Source: CAD feature listing. Evaluate the final solid. Frame: model axes, mm. Face numbers are marked on the shaded views. A direction names the side the tool comes from. Round coordinates to 2 decimals unless told otherwise and drop trailing zeros. Loops run counter-clockwise (first coordinate to the right, second up) from the corner with the lowest first, then second, coordinate; pieces in that order, holes last. Notation, with made-up numbers: (59.25, 36) -> (117.25, 36) arc R12 cw to (117.25, 52) -> close; hole circle Ø4 at (83.25, -29.75). An arc over 180 degrees is marked (long way). Write item = value, one per line.
from build123d import *

# Parameters (mm, degrees)
CYLINDER002_R               = 27.5
CYLINDER002_DEPTH           = 120
CYLINDER001_R               = 27.5
CYLINDER001_DEPTH           = 120
CYLINDER001_ROLL_ANGLE      = 89.363406
CYLINDER001_PITCH_ANGLE     = 89.363406
CYLINDER001_PLACEMENT_ANGLE = 90
CYLINDER_R                  = 27.5
CYLINDER_DEPTH              = 120
BOX001_W                    = 80
BOX001_H                    = 80
BOX001_DEPTH                = 80
BOX_W                       = 90
BOX_H                       = 90
BOX_DEPTH                   = 90


with BuildPart() as cylinder002:
    # Cylinder002 → Cylinder002 (new body)
    with BuildSketch(Plane.XZ.offset(-60)):
        Circle(CYLINDER002_R)
    extrude(amount=CYLINDER002_DEPTH)


with BuildPart() as cylinder001:
    # Cylinder001 → Cylinder001 (new body)
    with BuildSketch(Plane.XY):
        Circle(CYLINDER001_R)
    extrude(amount=CYLINDER001_DEPTH)


with BuildPart() as cylinder001_1:
    # Cylinder001 roll: moved
    add(cylinder001.part.rotate(Axis((0, 0, 0), (1, 0, 0)), CYLINDER001_ROLL_ANGLE))


with BuildPart() as cylinder001_2:
    # Cylinder001 pitch: moved
    add(cylinder001_1.part.rotate(Axis((0, 0, 0), (0, 1, 0)), CYLINDER001_PITCH_ANGLE))


with BuildPart() as cylinder001_3:
    # Cylinder001 placement: moved
    add(cylinder001_2.part.moved(Location((-60, 0, 0))).rotate(Axis((-60, 0, 0), (0, 0, 1)), CYLINDER001_PLACEMENT_ANGLE))


with BuildPart() as cylinder:
    # Cylinder → Cylinder (new body)
    with BuildSketch(Plane.XY.offset(-60)):
        Circle(CYLINDER_R)
    extrude(amount=CYLINDER_DEPTH)


with BuildPart() as cube001:
    # Box001 → Box001 (new body)
    with BuildSketch(Plane(origin=(-40, -40, -40), x_dir=(1, 0, 0), z_dir=(0, 0, 1))):
        with Locations((40, 40)):
            Rectangle(BOX001_W, BOX001_H)
    extrude(amount=BOX001_DEPTH)


with BuildPart() as cut003:
    # Box → Box (new body)
    with BuildSketch(Plane(origin=(-45, -45, -45), x_dir=(1, 0, 0), z_dir=(0, 0, 1))):
        with Locations((45, 45)):
            Rectangle(BOX_W, BOX_H)
    extrude(amount=BOX_DEPTH)

    # Cut: cut Cube001
    add(cube001.part, mode=Mode.SUBTRACT)

    # Cut001: cut Cylinder
    add(cylinder.part, mode=Mode.SUBTRACT)

    # Cut002: cut Cylinder001
    add(cylinder001_3.part, mode=Mode.SUBTRACT)

    # Cut003: cut Cylinder002
    add(cylinder002.part, mode=Mode.SUBTRACT)


solid = cut003.part
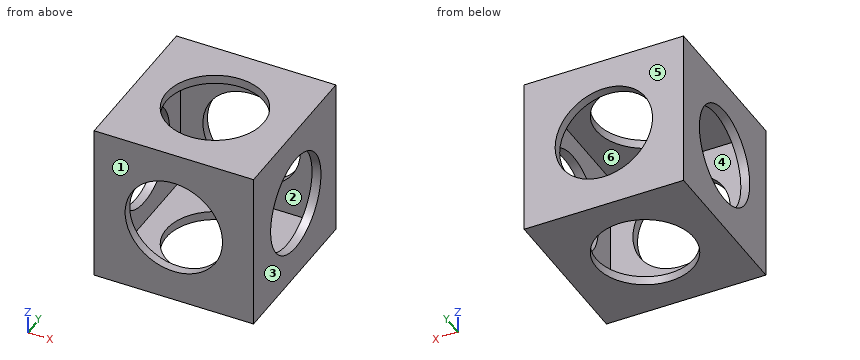
1. Section query B-B (y = 34). Return the cut outline in (x, z), then the cut area to 3 significant figures.
Evaluation:
outline = (-45, -45) -> (45, -45) -> (45, 45) -> (-45, 45) -> close; hole (-40, -40) -> (40, -40) -> (40, 40) -> (-40, 40) -> close
area = 1,700 mm²
2. Section query A-A (x = 0). Return the cut outline in (y, z), then the cut area to 3 significant figures.
Evaluation:
outline = (-45, -45) -> (-27.5, -45) -> (-27.5, -40) -> (-40, -40) -> (-40, -27.5) -> (-45, -27.5) -> close; (-45, 27.5) -> (-40, 27.5) -> (-40, 40) -> (-27.5, 40) -> (-27.5, 45) -> (-45, 45) -> close; (27.5, -45) -> (45, -45) -> (45, -27.5) -> (40, -27.5) -> (40, -40) -> (27.5, -40) -> close; (27.5, 40) -> (40, 40) -> (40, 27.5) -> (45, 27.5) -> (45, 45) -> (27.5, 45) -> close
area = 600 mm²
3. Set-up query: the marked faces 1 and 2. Return all of +Z, -Z, +X, -X, +Y, -Y with unobstructed straight access to the full face (end or side cutting, diameter ignored); none if empty.
Evaluation:
face_1 = +Z, -Z, +X, -X, -Y
face_2 = none
4. Mould query, pull axis Y, two halves, no side actions, for the marked faces 3, 4, 5 and 6. Classes: released by +Y, released by -Y, zero draft, split by the parting line, or undercut.
Evaluation:
face_3 = zero draft
face_4 = undercut
face_5 = released by +Y
face_6 = undercut
5. Line query: probe 1 along Y at (x, z) = (0, 43); probe 2 along X at (y, z) = (-36, -5.5). Output: solid intervals per line, ascending. Write a range as from..to.
Evaluation:
probe_1 = -45..-27.5, 27.5..45
probe_2 = -45..-40, 40..45
6. Section query D-D (z = 0). Give the number of separate pieces and of enclosed holes in the cut face, then the cut area to 3 significant figures.
Evaluation:
separate_pieces = 4
enclosed_holes = 0
area = 600 mm²
